from build123d import *

# Parameters (mm, degrees)
SKETCH2_R           = 2
SKETCH2_R_2         = 1.5
BOSS_EXTRUDE1_DEPTH = 2.45
SKETCH2_3_R         = 1.5
CUT_EXTRUDE1_DEPTH  = 3


with BuildPart() as part:
    # Sketch1 → Revolve1 (revolve)
    with BuildSketch(Plane.XY):
        with BuildLine():
            Line((0, -2.875), (0, 2.875))
            ThreePointArc((0, 2.875), (-2.875, 0), (0, -2.875))
        make_face()
    revolve(axis=Axis((0, 55, 0), (0, -1, 0)))

    # Sketch2 → Boss-Extrude1 (add, symmetric)
    with BuildSketch(Plane(origin=(0, 0, 0), x_dir=(1, 0, 0), z_dir=(0, 1, 0))):
        Circle(SKETCH2_R)
        Circle(SKETCH2_R_2, mode=Mode.SUBTRACT)
    extrude(amount=BOSS_EXTRUDE1_DEPTH, both=True)

    # Sketch2<3> → Cut-Extrude1 (cut, symmetric)
    with BuildSketch(Plane(origin=(0, 0, 0), x_dir=(1, 0, 0), z_dir=(0, 1, 0))):
        Circle(SKETCH2_3_R)
    extrude(amount=CUT_EXTRUDE1_DEPTH, both=True, mode=Mode.SUBTRACT)


solid = part.part
The model under review builds one solid part; all positions refer to its coordinate system, in mm. Round coordinates to 2 decimals unless told otherwise and drop trailing zeros. Loops run counter-clockwise (first coordinate to the right, second up) from the corner with the lowest first, then second, coordinate; pieces in that order, holes last. Notation, with made-up numbers: (59, -5.75) -> (91, -5.75) arc R16 cw to (91, 8.25) -> close; hole circle Ø10 at (38.5, 34.25). An arc over 180 degrees is marked (long way). Return JSON: item names as keys, results as strings.
(1) The part is to be moulded in two halves that separate along X. For faces 1 (the cylindrical face through (-0.325, 0.034, 1.464)), 2 (the cylindrical face through (-0.434, -2.255, 1.952)), say which applies: released by +X, released by -X, zero draft, split by the parting line, or undercut.
Solved:
{"face 1": "undercut", "face 2": "split by the parting line"}
(2) Add section C-C on x = 1.8. Write out the cut boundary in (y, z).
Solved:
{"outline": "(-2.45, -0.87) -> (-2.07, -0.87) arc R2.24 ccw to (2.07, -0.87) -> (2.45, -0.87) -> (2.45, 0.87) -> (2.07, 0.87) arc R2.24 ccw to (-2.07, 0.87) -> (-2.45, 0.87) -> close"}
(3) For pin 1 (1 mm diameter, centred on x = -2, z = 2, fed in from -Y); pin 2 (1.5 mm diameter, centred on x = 2, z = -1.5, fed in from -Y); pin 3 (1 mm diameter, centred on y = 0, z = -2, fed in from +X), all flat-tipped, find the tip position at first contact; note any pin that passes through.
Solved:
{"pin 1": "y = -1.69", "pin 2": "y = -2.45", "pin 3": "x = 2.45"}
(4) For line 1 (Y direction, x = 0.7, z = -1.5); line 2 (Z direction, x = 0.25, y = 0); line 3 (X direction, y = -0.05, z = 0), list the stretches that pass through material, from the lowest coordinate up.
Solved:
{"line 1": "-2.45 to 2.45", "line 2": "-2.86 to -1.48, 1.48 to 2.86", "line 3": "-2.87 to -1.5, 1.5 to 2.87"}
(5) Add section A-A on x = 0. Write out the cut boundary in (y, z) (3 decimals).
Solved:
{"outline": "(-2.453, -1.5) arc R2.875 ccw to (-2.45, -1.504) -> (-2.45, -2) -> (-2.065, -2) arc R2.875 ccw to (2.065, -2) -> (2.45, -2) -> (2.45, -1.504) arc R2.875 ccw to (2.453, -1.5) -> close; (-2.453, 1.5) -> (2.453, 1.5) arc R2.875 ccw to (2.45, 1.504) -> (2.45, 2) -> (2.065, 2) arc R2.875 ccw to (-2.065, 2) -> (-2.45, 2) -> (-2.45, 1.504) arc R2.875 ccw to start"}
(6) Add section B-B on z = 0. Write out the cut boundary in (x, y) (3 decimals), plus the area to 3 significant figures.
Solved:
{"outline": "(-2, -2.45) -> (-1.504, -2.45) arc R2.875 ccw to (-1.5, -2.453) -> (-1.5, 2.453) arc R2.875 ccw to (-1.504, 2.45) -> (-2, 2.45) -> (-2, 2.065) arc R2.875 ccw to (-2, -2.065) -> close; (1.5, -2.453) arc R2.875 ccw to (1.504, -2.45) -> (2, -2.45) -> (2, -2.065) arc R2.875 ccw to (2, 2.065) -> (2, 2.45) -> (1.504, 2.45) arc R2.875 ccw to (1.5, 2.453) -> close", "area": "9.89 mm2"}
(7) Add section D-D on z = -1.8. Write out the cut boundary in (x, y).
Solved:
{"outline": "(-0.87, -2.45) -> (0.87, -2.45) -> (0.87, -2.07) arc R2.24 ccw to (0.87, 2.07) -> (0.87, 2.45) -> (-0.87, 2.45) -> (-0.87, 2.07) arc R2.24 ccw to (-0.87, -2.07) -> close"}
